Geometry check sheet. Reference: the model listing, model coordinates, mm. A direction names the side the tool comes from. Round coordinates to 2 decimals unless told otherwise and drop trailing zeros. Write each loop counter-clockwise with the first axis right and the second up, starting at its lowest first coordinate (ties: lowest second). Pieces come first, ordered by that corner, then holes. Notation, with made-up numbers: (54, 26.25) -> (110, 26.25) arc R26 ccw to (110, 57.25) -> close; hole circle Ø1 at (86.5, 56.25). An arc over 180 degrees is marked (long way). One line per question, with ' | ' between items.
```python
from build123d import *

# Parameters (mm, degrees)
SKETCH1_R           = 50
BOSS_EXTRUDE1_DEPTH = 20
SKETCH2_R           = 25
BOSS_EXTRUDE2_DEPTH = 40
BOSS_EXTRUDE3_START = 20
SKETCH3_R           = 50
BOSS_EXTRUDE3_DEPTH = 20
SKETCH4_R           = 6
CUT_EXTRUDE1_DEPTH  = 107.77078252


with BuildPart() as part:
    # Sketch1 → Boss-Extrude1 (new body)
    with BuildSketch(Plane.XY):
        Circle(SKETCH1_R)
    extrude(amount=BOSS_EXTRUDE1_DEPTH)

    # Sketch2 → Boss-Extrude2 (add)
    with BuildSketch(Plane(origin=(0, 0, 0), x_dir=(-1, 0, 0), z_dir=(0, 0, -1))):
        Circle(SKETCH2_R)
    extrude(amount=BOSS_EXTRUDE2_DEPTH)

    # Sketch3 → Boss-Extrude3 (add)
    with BuildSketch(Plane(origin=(0, 0, -40), x_dir=(-1, 0, 0), z_dir=(0, 0, -1)).offset(BOSS_EXTRUDE3_START)):
        with Locations(Location((0, 0, 0), (0, 0, 180))):
            Circle(SKETCH3_R)
    extrude(amount=-BOSS_EXTRUDE3_DEPTH)

    # Sketch4 → Cut-Extrude1 (cut, through all)
    with BuildSketch(Plane.XY.offset(20)):
        Circle(SKETCH4_R)
    extrude(amount=-CUT_EXTRUDE1_DEPTH, mode=Mode.SUBTRACT)


solid = part.part
```
(1) Go/stop test with flat-tipped pins: pin 1 (12 mm diameter, centred on x = 32.5, z = -39, fed in from +Y); pin 2 (10 mm diameter, centred on x = -32, z = -26, fed in from -Y); pin 3 (14 mm diameter, centred on x = 0, y = 0, fed in from +Z); pin 4 (1 mm diameter, centred on x = -21, z = -15.5, fed in from -Y). Record where each tip stops, or that it passes through.
Resolved:
pin 1: stops at y = 42.35 | pin 2: passes through | pin 3: stops at z = 20 | pin 4: stops at y = -14.31
(2) Draft check along Y on faces 3 (the cylindrical face through (47.69, 15.02, 9.86)), 4 (the flat face through (-1, 10, -60)), 5 (the cylindrical face through (-6, 0, -19)). Enter one of: +Y half, -Y half, draft (parallel to the pull), parting line (faces both ways), or undercut.
Resolved:
face 3: parting line | face 4: draft | face 5: undercut
(3) Sectioned sample at C-C on z = -52. Record the cut outline in (x, y).
Resolved:
outline: circle Ø100 at (0, 0); hole circle Ø12 at (0, 0)
(4) Material ranges on line 1 (Z direction, x = -38, y = -23); line 2 (Y direction, x = 0, z = -36.5); line 3 (Y direction, x = 0, z = -43), recorded low to high.
Resolved:
line 1: z = -60 to -40, 0 to 20 | line 2: y = -25 to -6, 6 to 25 | line 3: y = -50 to -6, 6 to 50
(5) Sectioned sample at D-D on x = -18.5. Record the cut outline in (y, z), then the cut area to 3 significant figures.
Resolved:
outline: (-46.45, -60) -> (46.45, -60) -> (46.45, -40) -> (16.82, -40) -> (16.82, 0) -> (46.45, 0) -> (46.45, 20) -> (-46.45, 20) -> (-46.45, 0) -> (-16.82, 0) -> (-16.82, -40) -> (-46.45, -40) -> close | area: 5,060 mm2
(6) Sectioned sample at A-A on y = 0. Record the cut outline in (x, z).
Resolved:
outline: (-50, -60) -> (-6, -60) -> (-6, 20) -> (-50, 20) -> (-50, 0) -> (-25, 0) -> (-25, -40) -> (-50, -40) -> close; (6, -60) -> (50, -60) -> (50, -40) -> (25, -40) -> (25, 0) -> (50, 0) -> (50, 20) -> (6, 20) -> close
(7) Access from +Z, -Z, +X, -X, +Y, -Y to the whole of each face (thin tool, end or side, straight path). Record for faces 1 (the cylindrical face through (47.69, -15.02, -50.14)), 2 (the flat face through (-22.9, 10.4, -40)).
Resolved:
face 1: +Z, -Z | face 2: none
